```python
from build123d import *

# Parameters (mm, degrees)
BOSS_EXTRUDE1_DEPTH = 20
CHAMFER1_SIZE       = 2


with BuildPart() as part:
    # Sketch1 → Boss-Extrude1 (new body)
    with BuildSketch(Plane(origin=(0, 0, 0), x_dir=(1, 0, 0), z_dir=(0, 1, 0))):
        Polygon((42.830428459, 91.348139701), (18.601676139, 91.348139701), (-20, 57.741800753), (-20, 21.348139701), (0, 21.348139701), (0, 48.636252059), (26.0878441, 71.348139701), (42.830428459, 71.348139701), align=None)
    extrude(amount=BOSS_EXTRUDE1_DEPTH)

    # Chamfer1
    chamfer1_edges = [part.edges().sort_by_distance(p)[0] for p in [
        (-20, 0, -39.544970227),
        (-0.699161931, 0, -74.544970227),
        (30.716052299, 0, -91.348139701),
        (42.830428459, 0, -81.348139701),
        (-0.699161931, 20, -74.544970227),
        (-20, 20, -39.544970227),
        (-10, 20, -21.348139701),
        (0, 20, -34.99219588),
        (13.04392205, 20, -59.99219588),
        (34.459136279, 20, -71.348139701),
        (42.830428459, 20, -81.348139701),
        (34.459136279, 0, -71.348139701),
        (30.716052299, 20, -91.348139701),
        (13.04392205, 0, -59.99219588),
        (0, 0, -34.99219588),
        (-10, 0, -21.348139701),
    ]]
    chamfer(chamfer1_edges, length=CHAMFER1_SIZE)


solid = part.part
```
Here's how the part is built. I have some questions about the finished solid (model axes, mm). A direction names the side the tool comes from. Give positions to 0.01 mm unless a question says otherwise; leave off trailing zeros. Write each loop counter-clockwise with the first axis right and the second up, starting at its lowest first coordinate (ties: lowest second). Pieces come first, ordered by that corner, then holes.
(1) If I drill on L1, parallel to X at y = 8, z = -48.5; L2, parallel to Z at x = 28, y = 2.25; L3, parallel to X at y = 4.25, z = -67, over which ranges is the centre line in solid material (lowest first)?
Output values:
L1: x = -20 to 0
L2: z = -91.35 to -71.35
L3: x = -9.37 to 21.09
(2) Will these pins go through, and if not, where does the flat tip stop? pin 1 (12 mm diameter, centred on x = 8, y = 16.5, fed in from -Z); pin 2 (12 mm diameter, centred on x = 23.5, z = -63, fed in from -Y); pin 3 (6 mm diameter, centred on y = 7, z = -82.5, fed in from -X).
Output values:
pin 1: stops at z = -87.34
pin 2: stops at y = 0.6
pin 3: stops at x = 4.99
(3) On a 3-axis mill with a long thin cutter (end or side, diameter ignored), from which of +Z, -Z, +X, -X, +Y, -Y can I reach the whole of each face in a straight line? I mean faces 1 (the face through (33.96, 0.99, -72.36)), 2 (the face through (33.96, 19.01, -72.36)), 3 (the face through (0, 10, -35)). Say none if no direction works.
Output values:
face 1: +Z, +X, -Y
face 2: +Z, +X, +Y
face 3: +Z, +X, +Y, -Y
(4) Imagine slicing it at B-B, the plane z = -34.5. Write out the boundary of the cut face in (x, y), and give its area (3 significant figures).
Output values:
outline: (-20, 2) - (-18, 0) - (-2, 0) - (0, 2) - (0, 18) - (-2, 20) - (-18, 20) - (-20, 18) - close
area: 392 mm2
(5) Imagine slicing it at A-A, the plane y = 6. Write out the boundary of the cut face in (x, z), and give its area (3 significant figures).
Output values:
outline: (-20, -57.74) - (18.6, -91.35) - (42.83, -91.35) - (42.83, -71.35) - (26.09, -71.35) - (0, -48.64) - (0, -21.35) - (-20, -21.35) - close
area: 1,900 mm2
